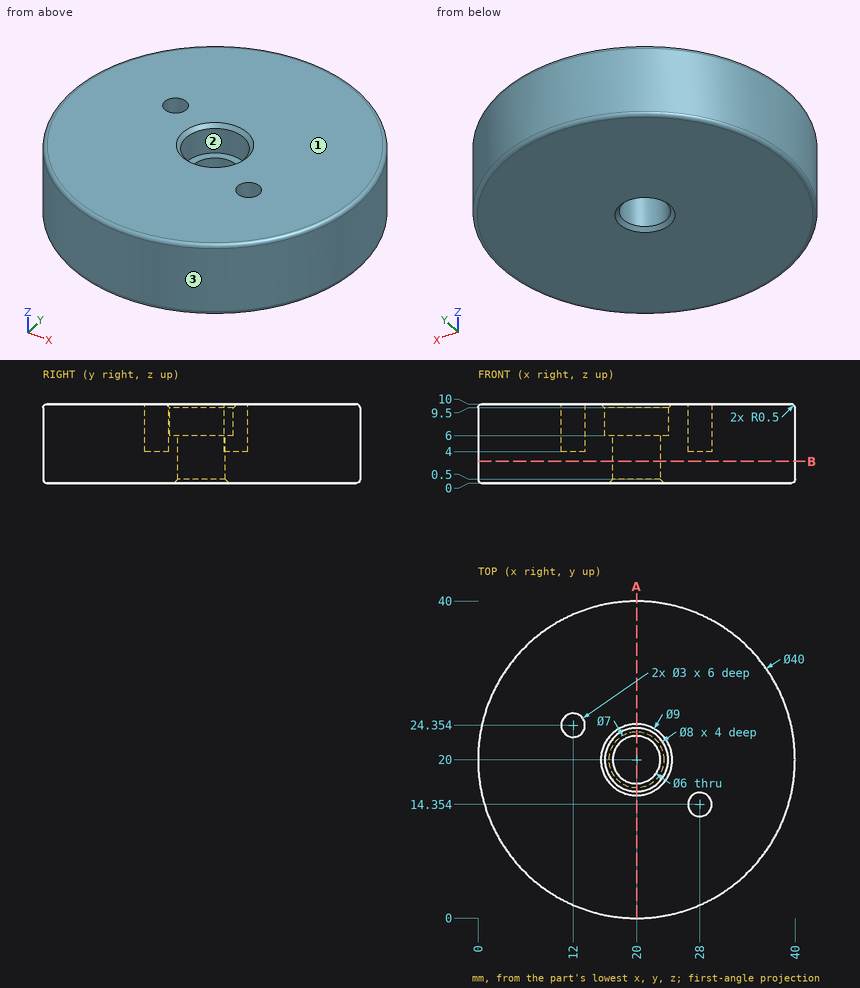
Drawing for the job (mm, zero at the part's lowest x, y, z). Coordinates: 2 decimals unless noted, no trailing zeros. Order: outer loops, then holes, each group sorted by start corner. A loop starts at its lowest first (then second) coordinate and runs counter-clockwise, first axis right, second up. Notation, with made-up numbers: (62, 67.5) -> (113, 67.5) arc R15 cw to (113, 93.5) -> close; hole circle Ø11 at (-5, 3). An arc over 180 degrees is marked (long way). Answer in a Markdown table with one row per item.
1) Mould opens along Y. For the marked faces 1, 2 and 3 say: pulls with the +Y half, pulls with the -Y half, needs draft (parallel to the pull), parting line crosses it, or undercut.
Check values:
| item | result |
|---|---|
| face 1 | needs draft |
| face 2 | undercut |
| face 3 | parting line crosses it |
2) Band-saw the part on A-A (x = 20). List the corners of the cut face in (y, z), and give its area (3 significant figures).
Check values:
| item | result |
|---|---|
| outline | (0, 0.5) arc R0.5 ccw to (0.5, 0) -> (16.5, 0) -> (17, 0.5) -> (17, 6) -> (16, 6) -> (16, 9.5) -> (15.5, 10) -> (0.5, 10) arc R0.5 ccw to (0, 9.5) -> close; (23, 0.5) -> (23.5, 0) -> (39.5, 0) arc R0.5 ccw to (40, 0.5) -> (40, 9.5) arc R0.5 ccw to (39.5, 10) -> (24.5, 10) -> (24, 9.5) -> (24, 6) -> (23, 6) -> close |
| area | 331 mm2 |
3) Drill centre lines: line 1 (X direction, y = 18.5, z = 8.5); line 2 (Y direction, x = 28, z = 8.1); line 3 (Y direction, x = 12, z = 8). Where is each one in solid material? Low to high.
Check values:
| item | result |
|---|---|
| line 1 | 0.06 to 16.29, 23.71 to 39.94 |
| line 2 | 1.67 to 12.85, 15.85 to 38.33 |
| line 3 | 1.67 to 22.85, 25.85 to 38.33 |
4) Band-saw the part on B-B (z = 2.75). List the corners of the cut face in (x, y), and give its area (3 significant figures).
Check values:
| item | result |
|---|---|
| outline | circle Ø40 at (20, 20); hole circle Ø6 at (20, 20) |
| area | 1,230 mm2 |
5) Flat gauge pins, fed straight in: P1, Ø3, axis at x = 28, z = 8.5, coming from the +Y side; P2, Ø1.5, axis at x = 5, z = 8.5, coming from the -Y side; P3, Ø0.9, axis at x = 28, y = 14, coming from the +Z side. Where does each tip first touch, or does it go through?
Check values:
| item | result |
|---|---|
| P1 | y = 38.91 |
| P2 | y = 5.97 |
| P3 | z = 4 |
